The figure shows three views and two pictorial views of one solid part (mm, origin at its lowest corner). Answer the questions. Coordinates: 2 decimals unless noted, no trailing zeros. Order: outer loops, then holes, each group sorted by start corner. A loop starts at its lowest first (then second) coordinate and runs counter-clockwise, first axis right, second up. Notation, with made-up numbers: M -18.5,43.25 L -2.5,43.25 A20 cw -2.5,74.25 Z; hole C 39.25,-27.5 d9. An arc over 180 degrees is marked long. Answer in a Markdown table with one row per item. Add a question column.
Item 1: The part is cut by section B-B (y = 14.5). State how many separate pieces and enclosed holes the cut face has.
Item 2: Flat-ended cylindrical pins translate along their axes: pin 1 Ø1.6 at (x, z) = (8, 2) entering from +Y; pin 2 Ø1 at (y, z) = (10, 2) entering from +X (1 decimal); pin 3 Ø1 at (x, z) = (74.5, 1) entering from -Y; pin 4 Ø1.5 at (x, y) = (83, 43) entering from -Z. Find the tip coordinate at first contact, or state that the pin passes through.
Item 3: Consider line 1 (X direction, y = 42, z = 1.15) (1 decimal); line 2 (X direction, y = 21.5, z = 1.75); line 3 (Y direction, x = 155, z = 0.85). Determine where each line is inside the solid, lowest interval first. Write a range as from..to.
Item 4: The part is cut by section A-A (y = 40). Write down the section's boundary in (x, z) (1 decimal).
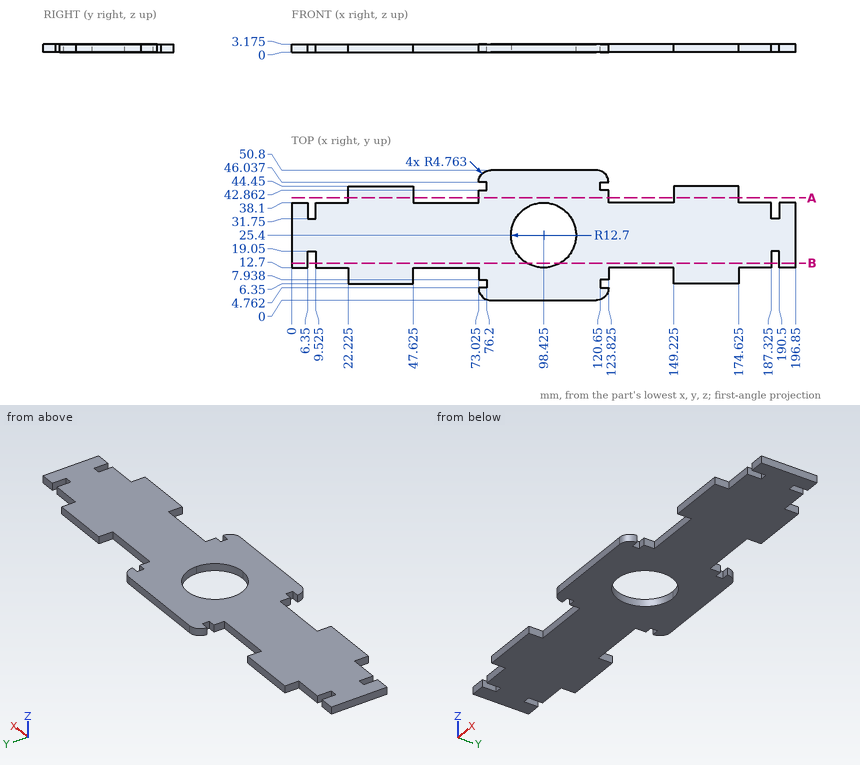
Reply:
| question | item | result |
|---|---|---|
| 1 | separate pieces | 4 |
| 1 | enclosed holes | 0 |
| 2 | pin 1 | stops at y = 31.75 |
| 2 | pin 2 | stops at x = 174.6 |
| 2 | pin 3 | stops at y = 0.9 |
| 2 | pin 4 | stops at z = 0 |
| 3 | line 1 | x = 22.2..47.6, 73..123.8, 149.2..174.6 |
| 3 | line 2 | x = 0..86.34, 110.51..196.85 |
| 3 | line 3 | y = 6.35..44.45 |
| 4 | outline | M 22.2,0 L 47.6,0 L 47.6,3.2 L 22.2,3.2 Z; M 73,0 L 123.8,0 L 123.8,3.2 L 73,3.2 Z; M 149.2,0 L 174.6,0 L 174.6,3.2 L 149.2,3.2 Z |
